Model file for the job. Use its own axes, mm. A direction names the side the tool comes from. Give positions to 0.01 mm unless a question says otherwise; leave off trailing zeros. Loops run counter-clockwise (first coordinate to the right, second up) from the corner with the lowest first, then second, coordinate; pieces in that order, holes last. Notation, with made-up numbers: M 72.5,77 L 109.5,77 A17 cw 109.5,99 Z; hole C 32.5,25.25 d10. An arc over 180 degrees is marked long. Answer in a Markdown table with one row per item.
```python
from build123d import *

# Parameters (mm, degrees)
SKETCH1_R                 = 4.5
MAIN_BASE_DEPTH           = 3
MOTOR_SHAFT_CUT_OUT_DEPTH = 8.03562364


with BuildPart() as part:
    # Sketch1 → main_base (new body)
    with BuildSketch(Plane.XY):
        Circle(SKETCH1_R)
    extrude(amount=MAIN_BASE_DEPTH)

    # Sketch2 → pulley_cut_out (revolve, cut)
    with BuildSketch(Plane(origin=(0, 0, 0), x_dir=(0, 0, -1), z_dir=(1, 0, 0)), mode=Mode.PRIVATE) as pulley_cut_out_sk:
        Polygon((-2.5, 4.5), (-0.5, 4.5), (-1, 4), (-2, 4), align=None)
    revolve(pulley_cut_out_sk.sketch.rotate(Axis((0, 0, 0), (0, 0, 1)), 90), axis=Axis((0, 0, 0), (0, 0, 1)), mode=Mode.SUBTRACT)

    # Sketch3 → motor_shaft_cut_out (cut, through all)
    with BuildSketch(Plane.XY):
        with BuildLine():
            ThreePointArc((1.205, 0), (1.127652187, 0.424765283), (0.905538514, 0.795))
            Line((0.905538514, 0.795), (-0.905538514, 0.795))
            ThreePointArc((-0.905538514, 0.795), (-0.424765283, -1.127652187), (1.205, 0))
        make_face()
    extrude(amount=MOTOR_SHAFT_CUT_OUT_DEPTH, mode=Mode.SUBTRACT)


solid = part.part
```
Q1. Drop flat-ended pins along their axis: pin 1 (1.4 mm diameter, centred on x = -0.5, z = 1, fed in from -Y); pin 2 (1 mm diameter, centred on y = -1, z = 0.5, fed in from +X). Give the stop position or say it passes through.
Reported:
| item | result |
|---|---|
| pin 1 | y = -4.5 |
| pin 2 | x = 4.47 |
Q2. Saw through at C-C (z = 2.65). Give the cut face in (x, y) (3 decimals), and give its area (3 significant figures).
Reported:
| item | result |
|---|---|
| outline | C 0,0 d9; hole M -0.906,0.795 A1.205 ccw long 0.906,0.795 Z |
| area | 59.6 mm² |
Q3. Mould opens along Z. For faces 1 (the face through (0, 1, 0)), 2 (the face through (-0.59, 4.46, 2.75)), 3 (the face through (0.867, 3.905, 1.507)) say: released by +Z, released by -Z, zero draft, split by the parting line, or undercut.
Reported:
| item | result |
|---|---|
| face 1 | released by -Z |
| face 2 | zero draft |
| face 3 | undercut |
Q4. 3-axis set-ups, long thin cutter, end or side, ignore diameter. For faces 4 (the face through (0, 0.795, 1)), 5 (the face through (0, 1, 3)): which of +Z, -Z, +X, -X, +Y, -Y reach the whole face in a straight line?
Reported:
| item | result |
|---|---|
| face 4 | +Z, -Z |
| face 5 | +Z, +X, -X, +Y, -Y |
Q5. Probe probe 1 along Y at (x, z) = (0, 1.5) (3 decimals); probe 2 along Z at (x, y) = (-0.5, -4); probe 3 along X at (y, z) = (-0.75, 1.6). List the from-to ranges inside material, lowest first.
Reported:
| item | result |
|---|---|
| probe 1 | -4 to -1.205, 0.795 to 4 |
| probe 2 | 0 to 0.97, 2.03 to 3 |
| probe 3 | -3.93 to -0.94, 0.94 to 3.93 |
Q6. Saw through at A-A (x = 0). Give the cut face in (y, z) (3 decimals).
Reported:
| item | result |
|---|---|
| outline | M -4.5,0 L -1.205,0 L -1.205,3 L -4.5,3 L -4.5,2.5 L -4,2 L -4,1 L -4.5,0.5 Z; M 0.795,0 L 4.5,0 L 4.5,0.5 L 4,1 L 4,2 L 4.5,2.5 L 4.5,3 L 0.795,3 Z |
Q7. Saw through at B-B (z = 1.6). Give the cut face in (x, y) (3 decimals), and give its area (3 significant figures).
Reported:
| item | result |
|---|---|
| outline | C 0,0 d8; hole M -0.906,0.795 A1.205 ccw long 0.906,0.795 Z |
| area | 46.2 mm² |
